```python
from build123d import *

# Parameters (mm, degrees)
F1_DEPTH = 12
F2_R     = 2.5
F3_DEPTH = 4
F4_W     = 6
F4_H     = 12
F4_R     = 1.5
F5_DEPTH = 3
F6_DEPTH = 6.5712102501


with BuildPart() as f1:
    # F0 (on Top) → F1 (new body)
    with BuildSketch(Plane.XY):
        Polygon((-20, -5), (-20, 0), (0, 0), (0, -5), (5, -5), (5, 83.330666624), (0, 83.330666624), (-25, 0), (-25, -5), align=None)
        Polygon((1, 4), (-19.6238279597, 4), (1, 72.743893289), align=None, mode=Mode.SUBTRACT)
    extrude(amount=F1_DEPTH)

    # F2 (on face) → F3 (cut, through all)
    with BuildSketch(Plane.XZ):
        with Locations((-10, 6)):
            Circle(F2_R)
    extrude(amount=-F3_DEPTH, mode=Mode.SUBTRACT)

    # F4 (on face) → F5 (join)
    with BuildSketch(Plane(origin=(-22.9356586075, 6.8809177751, 0), x_dir=(-0.2873563218, -0.9578237543, 0), z_dir=(-0.9578237543, 0.2873563218, 0))):
        with Locations((-76.816091954, 6)):
            Rectangle(F4_W, F4_H)
        with Locations((-76.816091954, 6)):
            Circle(F4_R, mode=Mode.SUBTRACT)
        with Locations((-11.816091954, 6)):
            Rectangle(F4_W, F4_H)
        with Locations((-11.816091954, 6)):
            Circle(F4_R, mode=Mode.SUBTRACT)
    extrude(amount=F5_DEPTH)

    # F4 (on face) → F6 (cut, through all)
    with BuildSketch(Plane(origin=(-22.9356586075, 6.8809177751, 0), x_dir=(-0.2873563218, -0.9578237543, 0), z_dir=(-0.9578237543, 0.2873563218, 0))):
        with Locations((-76.816091954, 6)):
            Circle(F4_R)
        with Locations((-11.816091954, 6)):
            Circle(F4_R)
    extrude(amount=-F6_DEPTH, mode=Mode.SUBTRACT)


solid = f1.part
```
Geometry check sheet. Reference: the model listing, model coordinates, mm. A direction names the side the tool comes from. Coordinates: 2 decimals unless noted, no trailing zeros. Write each loop counter-clockwise with the first axis right and the second up, starting at its lowest first coordinate (ties: lowest second). Pieces come first, ordered by that corner, then holes. Notation, with made-up numbers: M -36,-7 L -32,-7 A25 cw -32,29 Z; hole C 14.5,17 d6. An arc over 180 degrees is marked long. One line per item, written item: value. Start each with the question number.
(1) Sectioned sample at B-B, the plane x = -10. Enter the section's corners in (y, z).
(2) Sectioned sample at C-C, the plane y = 13. Enter the section's corners in (x, z).
(3) Release check for a two-part mould opening along Z. For faces 4 (the face through (-10.24, 35.86, 12)), 5 (the face through (-7, 4, 6)), 6 (the face through (-11.84, 1.97, 7.69)) record: released by +Z, released by -Z, zero draft, split by the parting line, or undercut.
(4) Scan lines: line 1 along Z through (x, y) = (-10, 2.1); line 2 along Y through (x, z) = (1.5, 1); line 3 along X through (y, z) = (47.5, 4). Record each from-to range of solid material in increasing order. Write a range as [from, to].
(5) Tool access check on faces 1 (the face through (-3.14, 78.01, 5.92)), 2 (the face through (-9.456, 37.891, 5.916)), 3 (the face through (3, 83.331, 6)). Record the directions out of +Z, -Z, +X, -X, +Y, -Y that give a thin tool (end or side, any length) a straight path to the whole face; none if there is none.
(6) Depth check by flat-ended pin: pin 1 (2 mm diameter, centred on x = -16, z = 3, fed in from -Y); pin 2 (5.5 mm diameter, centred on x = 1.5, z = 3.5, fed in from +Y); pin 3 (6 mm diameter, centred on y = 51, z = 5, fed in from -X). Enter the tip coordinate at first touch or a pass-through.
(7) Sectioned sample at A-A, the plane z = 6. State how many separate pieces and enclosed holes the cut face has, and give its area (3 significant figures).
Filled sheet:
1. outline: M 0,0 L 4,0 L 4,3.5 L 0,3.5 Z; M 0,8.5 L 4,8.5 L 4,12 L 0,12 Z; M 36.08,0 L 50,0 L 50,12 L 36.08,12 Z
2. outline: M -21.1,0 L -16.92,0 L -16.92,12 L -21.1,12 Z; M 1,0 L 5,0 L 5,12 L 1,12 Z
3. face 4: released by +Z
3. face 5: zero draft
3. face 6: undercut
4. line 1: [0, 3.5], [8.5, 12]
4. line 2: [-5, 83.33]
4. line 3: [-10.75, -6.57], [1, 5]
5. face 1: +Z, -Z, -X
5. face 2: +Z, -Z
5. face 3: +Z, -Z, +X, +Y
6. pin 1: y = 0
6. pin 2: y = 83.71
6. pin 3: x = -10.6
7. separate pieces: 3
7. enclosed holes: 0
7. area: 767 mm²
